Answer from the drawing. Dimensions are ordinates in mm from the lowest x, y and z of the part. A direction names the side the tool comes from. Round coordinates to 2 decimals unless told otherwise and drop trailing zeros. Loops run counter-clockwise (first coordinate to the right, second up) from the corner with the lowest first, then second, coordinate; pieces in that order, holes last. Notation, with made-up numbers: (-21, -26) - (1, -26) arc R8 ccw to (1, -22) - close; hole circle Ø10 at (37, 56). An arc over 180 degrees is marked (long way). Answer as CSV lines item,"result". Start each with the question number.
Q1. The mould has two halves that part along Y. Classify the marked faces 1, 2 and 3: +Y half, -Y half, draft (parallel to the pull), parting line (faces both ways), or undercut.
Q2. Straight lines are drawn through the part: L1, parallel to Y at x = 50, z = 11.25; L2, parallel to Z at x = 27, y = 57.5; L3, parallel to Y at x = 33.5, z = 12. For each, find the intervals that lie inside material, in ascending order. Write a range as [from, to].
Q3. Section A-A on y = 50 is taken. Write down the section's boundary in (x, z).
Q4. For the marked faces 4 and 5, determine the directions among +Z, -Z, +X, -X, +Y, -Y from which every point of the face is accessible in a straight line to the end or side of a thin tool.
Q5. Section B-B on x = 50 is taken. Write down the section's boundary in (y, z).
Q6. Each of these flat-tipped pins is pushed along its axis until it touches: pin 1 Ø8 at (y, z) = (27.5, 7.5) entering from -X; pin 2 Ø6 at (x, z) = (61, 11.5) entering from -Y; pin 3 Ø8 at (x, y) = (20, 87.5) entering from -Z; pin 4 Ø9 at (x, y) = (50, 67.45) entering from +Z. Where does it stop, or does it pass through?
Q7. Section C-C on z = 5 is taken. Write down the section's boundary in (x, y).
Q8. Section D-D on x = 65 is taken. Write down the section's boundary in (y, z).
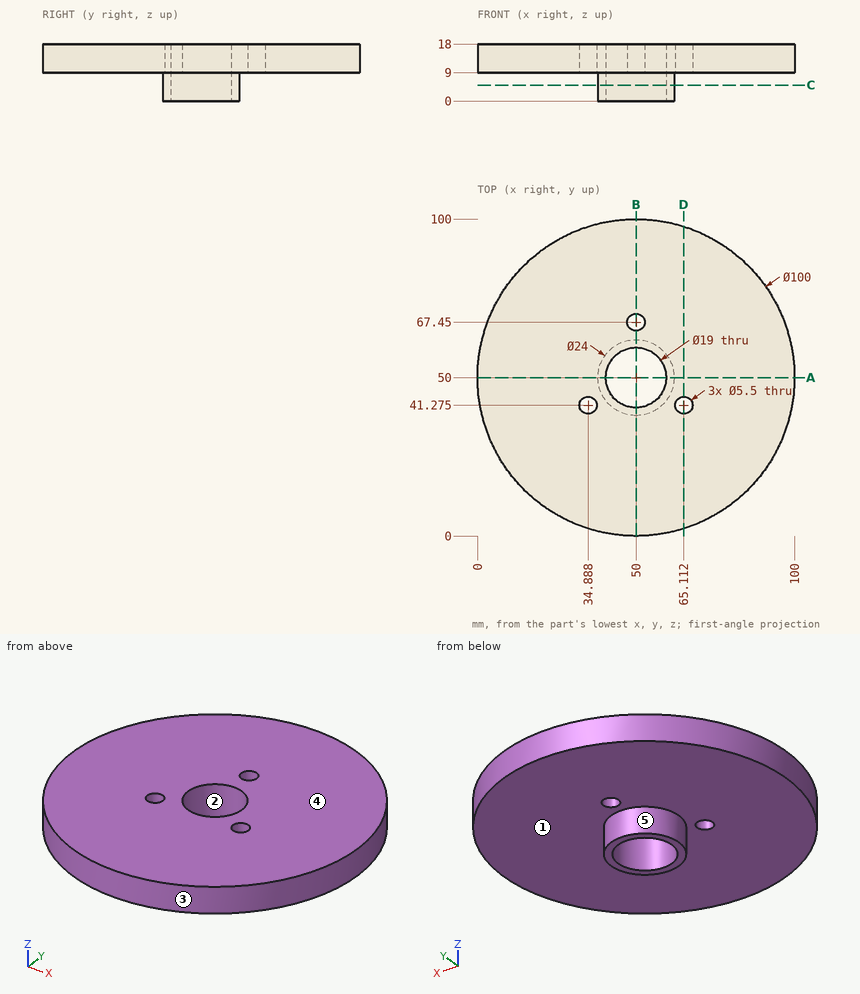
Findings:
1,face 1,"draft"
1,face 2,"undercut"
1,face 3,"parting line"
2,L1,"y = [0, 40.5], [59.5, 64.7], [70.2, 100]"
2,L2,"z = [9, 18]"
2,L3,"y = [2.8, 38.9], [43.65, 97.2]"
3,outline,"(0, 9) - (38, 9) - (38, 0) - (40.5, 0) - (40.5, 18) - (0, 18) - close; (59.5, 0) - (62, 0) - (62, 9) - (100, 9) - (100, 18) - (59.5, 18) - close"
4,face 4,"+Z, +X, -X, +Y, -Y"
4,face 5,"-Z"
5,outline,"(0, 9) - (38, 9) - (38, 0) - (40.5, 0) - (40.5, 18) - (0, 18) - close; (59.5, 0) - (62, 0) - (62, 9) - (64.7, 9) - (64.7, 18) - (59.5, 18) - close; (70.2, 9) - (100, 9) - (100, 18) - (70.2, 18) - close"
6,pin 1,"stops at x = 3.67"
6,pin 2,"stops at y = 0.64"
6,pin 3,"stops at z = 9"
6,pin 4,"stops at z = 18"
7,outline,"circle Ø24 at (50, 50); hole circle Ø19 at (50, 50)"
8,outline,"(2.3, 9) - (38.53, 9) - (38.53, 18) - (2.3, 18) - close; (44.02, 9) - (97.7, 9) - (97.7, 18) - (44.02, 18) - close"
